Part model, mm, in its own coordinate system. A direction names the side the tool comes from. Round coordinates to 2 decimals unless told otherwise and drop trailing zeros. Loops run counter-clockwise (first coordinate to the right, second up) from the corner with the lowest first, then second, coordinate; pieces in that order, holes last. Notation, with made-up numbers: (79.25, -4) -> (138.25, -4) arc R17 ccw to (138.25, 10) -> close; hole circle Ø1 at (1.5, 34.5). An arc over 180 degrees is marked (long way). Answer as CSV lines item,"result".
from build123d import *

# Parameters (mm, degrees)
F0_R     = 25.4
F0_W     = 25.4
F0_H     = 25.4
F1_DEPTH = 2.54
F2_R     = 25.4
F2_R_2   = 24.13
F2_W     = 27.94
F2_H     = 27.94
F2_W_2   = 25.4
F2_H_2   = 25.4
F3_DEPTH = 1.27
F4_R     = 25.4
F4_R_2   = 24.13
F4_W     = 27.94
F4_H     = 27.94
F4_W_2   = 25.4
F4_H_2   = 25.4
F5_DEPTH = 1.27


with BuildPart() as f1:
    # F0 (on Top) → F1 (new body)
    with BuildSketch(Plane.XY):
        Circle(F0_R)
        Rectangle(F0_W, F0_H, mode=Mode.SUBTRACT)
    extrude(amount=F1_DEPTH)

    # F2 (on face) → F3 (join)
    with BuildSketch(Plane.XY.offset(2.54)):
        Circle(F2_R)
        Circle(F2_R_2, mode=Mode.SUBTRACT)
        Rectangle(F2_W, F2_H)
        Rectangle(F2_W_2, F2_H_2, mode=Mode.SUBTRACT)
    extrude(amount=F3_DEPTH)

    # F4 (on face) → F5 (join)
    with BuildSketch(Plane(origin=(0, 0, 0), x_dir=(1, 0, 0), z_dir=(0, 0, -1))):
        Circle(F4_R)
        Circle(F4_R_2, mode=Mode.SUBTRACT)
        Rectangle(F4_W, F4_H)
        Rectangle(F4_W_2, F4_H_2, mode=Mode.SUBTRACT)
    extrude(amount=F5_DEPTH)


solid = f1.part
Q1. Two-plate mould, pull along X, no slides. Class faces 6 (the face through (22.5, 9.3, -1.27)), 7 (the face through (0, 12.7, 1)), 8 (the face through (-5.506, 24.796, 1.306)), 9 (the face through (0, -16, 2.54)): pulls with the +X half, pulls with the -X half, needs draft (parallel to the pull), parting line crosses it, or undercut.
Geometry results:
face 6,"needs draft"
face 7,"undercut"
face 8,"parting line crosses it"
face 9,"undercut"
Q2. Which spindle directions (+Z, -Z, +X, -X, +Y, -Y) get a long thin tool onto all of the face, cutting with end or side? Do faces 1 (the face through (-13.97, 0, -1)), 2 (the face through (-1, 13, -1.27)), 3 (the face through (13.97, 0, 3)), 4 (the face through (0, -12.7, 1)), 5 (the face through (22.5, -9.3, 3.81)). Say none if no direction does.
Geometry results:
face 1,"-Z"
face 2,"-Z, +X, -X, +Y, -Y"
face 3,"+Z"
face 4,"+Z, -Z"
face 5,"+Z, +X, -X, +Y, -Y"
Q3. Drop flat-ended pins along their axis: P1, Ø0.6, axis at y = 6, z = -1, coming from the +X side; P2, Ø1.5, axis at x = -18, y = -8.5, coming from the -Z side; P3, Ø3, axis at x = 9.5, y = 6.5, coming from the +Z side; P4, Ø1, axis at y = -4, z = -1, coming from the -X side. Give the stop position or say it passes through.
Geometry results:
P1,"x = 24.75"
P2,"z = 0"
P3,"through"
P4,"x = -25.16"
Q4. Drill centre lines: line 1 along X through (y, z) = (0, -0.65); line 2 along X through (y, z) = (-11, 2.6). Where is each one in solid material? Low to high.
Geometry results:
line 1,"-25.4 to -24.13, -13.97 to -12.7, 12.7 to 13.97, 24.13 to 25.4"
line 2,"-22.89 to -21.48, -13.97 to -12.7, 12.7 to 13.97, 21.48 to 22.89"
Q5. Saw through at C-C, the plane x = 20.5. Write the cut outline in (y, z).
Geometry results:
outline,"(-15, -1.27) -> (-12.73, -1.27) -> (-12.73, 0) -> (12.73, 0) -> (12.73, -1.27) -> (15, -1.27) -> (15, 3.81) -> (12.73, 3.81) -> (12.73, 2.54) -> (-12.73, 2.54) -> (-12.73, 3.81) -> (-15, 3.81) -> close"
Q6. Saw through at A-A, the plane x = 0. Write the cut outline in (y, z).
Geometry results:
outline,"(-25.4, -1.27) -> (-24.13, -1.27) -> (-24.13, 0) -> (-13.97, 0) -> (-13.97, -1.27) -> (-12.7, -1.27) -> (-12.7, 3.81) -> (-13.97, 3.81) -> (-13.97, 2.54) -> (-24.13, 2.54) -> (-24.13, 3.81) -> (-25.4, 3.81) -> close; (12.7, -1.27) -> (13.97, -1.27) -> (13.97, 0) -> (24.13, 0) -> (24.13, -1.27) -> (25.4, -1.27) -> (25.4, 3.81) -> (24.13, 3.81) -> (24.13, 2.54) -> (13.97, 2.54) -> (13.97, 3.81) -> (12.7, 3.81) -> close"
Q7. Saw through at D-D, the plane y = 16.5. Write the cut outline in (x, z).
Geometry results:
outline,"(-19.31, -1.27) -> (-17.61, -1.27) -> (-17.61, 0) -> (17.61, 0) -> (17.61, -1.27) -> (19.31, -1.27) -> (19.31, 3.81) -> (17.61, 3.81) -> (17.61, 2.54) -> (-17.61, 2.54) -> (-17.61, 3.81) -> (-19.31, 3.81) -> close"
